```python
from build123d import *

# Parameters (mm, degrees)
F0_W     = 101.6
F0_H     = 50.8
F1_DEPTH = 25.4
F2_R     = 6.35
F3_DEPTH = 25.401
F4_W     = 12.7
F4_H     = 25.4
F6_W     = 10.16
F6_H     = 6.35
F8_R     = 1.27
F9_SIZE  = 2.54


with BuildPart() as f1:
    # F0 (on Front) → F1 (new body)
    with BuildSketch(Plane.XZ):
        Rectangle(F0_W, F0_H)
    extrude(amount=F1_DEPTH)

    # F2 (on face) → F3 (cut, through all)
    with BuildSketch(Plane.XZ.offset(25.4)):
        with Locations((-38.1, 12.7)):
            Circle(F2_R)
        with Locations((-38.1, -12.7)):
            Circle(F2_R)
        with Locations((38.1, -12.7)):
            Circle(F2_R)
        with Locations((38.1, 12.7)):
            Circle(F2_R)
    extrude(amount=-F3_DEPTH, mode=Mode.SUBTRACT)

    # F4 (on Top) → F5 (revolve)
    with BuildSketch(Plane.XY):
        with Locations((-6.35, 12.7)):
            Rectangle(F4_W, F4_H)
    revolve(axis=Axis((0, 12.7, 0), (0, 1, 0)))

    # F6 (on Top) → F7 (revolve, cut)
    with BuildSketch(Plane.XY):
        with Locations((-13.302147, 13.335)):
            Rectangle(F6_W, F6_H)
    revolve(axis=Axis((0, 12.941601, 0), (0, 1, 0)), mode=Mode.SUBTRACT)

    # F8
    f8_edges = [f1.edges().sort_by_distance(p)[0] for p in [
        (12.7, 0, 0),
        (8.222147, 10.16, 0),
        (8.222147, 16.51, 0),
    ]]
    fillet(f8_edges, radius=F8_R)

    # F9
    f9_edges = [f1.edges().sort_by_distance(p)[0] for p in [
        (0, 0, -25.4),
        (-50.8, 0, 0),
        (0, 0, 25.4),
        (50.8, 0, 0),
    ]]
    chamfer(f9_edges, length=F9_SIZE)


solid = f1.part
```
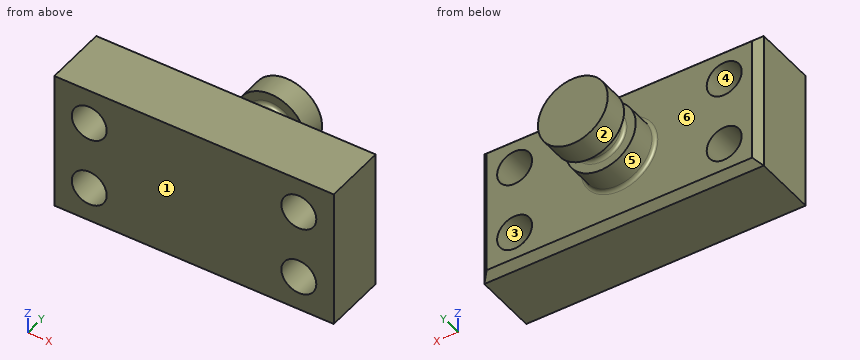
Geometry: final body of the model. Coordinates: model frame, mm. Face numbers are marked on the shaded views. A direction names the side the tool comes from. Coordinates: 2 decimals unless noted, no trailing zeros. Order: outer loops, then holes, each group sorted by start corner. A loop starts at its lowest first (then second) coordinate and runs counter-clockwise, first axis right, second up. Notation, with made-up numbers: (50, 51) - (99, 51) arc R10 cw to (99, 64) - close; hole circle Ø3 at (46, -8). An arc over 180 degrees is marked (long way). Write each question's results on one line, items separated by ' | '.
1) Line query: line 1 (Z direction, x = 38.1, y = -11.25); line 2 (X direction, y = -8, z = -12); line 3 (Y direction, x = 10, z = 4). Output: solid intervals per line, ascending. Write a range as from..to.
Results list:
line 1: -25.4..-19.05, -6.35..6.35, 19.05..25.4 | line 2: -50.8..-44.41, -31.79..31.79, 44.41..50.8 | line 3: -25.4..10.16, 16.51..25.4
2) Section B-B, the plane y = -8. Return loops of the section in (x, z).
Results list:
outline: (-50.8, -25.4) - (50.8, -25.4) - (50.8, 25.4) - (-50.8, 25.4) - close; hole circle Ø12.7 at (-38.1, -12.7); hole circle Ø12.7 at (-38.1, 12.7); hole circle Ø12.7 at (38.1, -12.7); hole circle Ø12.7 at (38.1, 12.7)
3) Section A-A, the plane x = -38.1. Return loops of the section in (y, z), plus the area to 3 significant figures.
Results list:
outline: (-25.4, -25.4) - (-2.54, -25.4) - (0, -22.86) - (0, -19.05) - (-25.4, -19.05) - close; (-25.4, -6.35) - (0, -6.35) - (0, 6.35) - (-25.4, 6.35) - close; (-25.4, 19.05) - (0, 19.05) - (0, 22.86) - (-2.54, 25.4) - (-25.4, 25.4) - close | area: 639 mm^2
4) Section C-C, the plane x = 0. Return loops of the section in (y, z), plus the area to 3 significant figures.
Results list:
outline: (-25.4, -25.4) - (-2.54, -25.4) - (0, -22.86) - (0, -13.97) arc R1.27 cw to (1.27, -12.7) - (10.16, -12.7) - (10.16, -9.49) arc R1.27 cw to (11.43, -8.22) - (15.24, -8.22) arc R1.27 cw to (16.51, -9.49) - (16.51, -12.7) - (25.4, -12.7) - (25.4, 12.7) - (16.51, 12.7) - (16.51, 9.49) arc R1.27 cw to (15.24, 8.22) - (11.43, 8.22) arc R1.27 cw to (10.16, 9.49) - (10.16, 12.7) - (1.27, 12.7) arc R1.27 cw to (0, 13.97) - (0, 22.86) - (-2.54, 25.4) - (-25.4, 25.4) - close | area: 1,870 mm^2
5) Set-up query: the marked faces 1 and 2. Return all of +Z, -Z, +X, -X, +Y, -Y with unobstructed straight access to the full face (end or side cutting, diameter ignored); none if empty.
Results list:
face 1: +Z, -Z, +X, -X, -Y | face 2: +Y
6) Pull-direction query (Z, two-part tool) for the marked faces 3, 4, 5 and 6; classes: pulls with the +Z half, pulls with the -Z half, needs draft (parallel to the pull), parting line crosses it, or undercut.
Results list:
face 3: undercut | face 4: undercut | face 5: parting line crosses it | face 6: needs draft
7) Section D-D, the plane z = 20.5. Return loops of the section in (x, y), plus the area to 3 significant figures.
Results list:
outline: (-50.8, -25.4) - (50.8, -25.4) - (50.8, -2.54) - (48.26, 0) - (-48.26, 0) - (-50.8, -2.54) - close | area: 2,570 mm^2
8) Pin query (flat end, axial travel): pin 1 (5 mm diameter, centred on x = -16.5, z = -14.5, fed in from +Y); pin 2 (10 mm diameter, centred on y = 19, z = -18, fed in from +X); pin 3 (6 mm diameter, centred on x = 10.5, y = 7.5, fed in from -Z). Return the tip coordinate at first contact, or that it passes through.
Results list:
pin 1: y = 0 | pin 2: through | pin 3: z = -10.25
